Read the model definition and answer for the solid it produces. Units are mm, in the model's axes. A direction names the side the tool comes from. Give positions to 0.01 mm unless a question says otherwise; leave off trailing zeros. Loops run counter-clockwise (first coordinate to the right, second up) from the corner with the lowest first, then second, coordinate; pieces in that order, holes last.
(1) Find section A-A, the plane y = -16. Write down the section's boundary in (x, z), then the cut area to 3 significant figures.
(2) Find section B-B, the plane z = 2. Write down the section's boundary in (x, y).
(3) Determine the mould class of faces 1 (the face through (5, -5, 5)), 2 (the face through (-1, -10, 40)), 3 (the face through (-27, -20, 1)) for opening direction Z: pulls with the +Z half, pulls with the -Z half, needs draft (parallel to the pull), parting line crosses it, or undercut.
(4) Which of the six approach directions +Z, -Z, +X, -X, +Y, -Y give full straight-line access (tool end or side, diameter ignored) to faces 4 (the face through (-32, -5, -20)), 5 (the face through (-1, 0, 1))?
(5) Find section D-D, the plane y = -6.5. Write down the section's boundary in (x, z), then the cut area to 3 significant figures.
(6) Find section C-C, the plane x = -32. Write down the section's boundary in (y, z).
(7) This flat-tipped pin is pushed along its axis until it touches: P1, Ø2.5, axis at x = -33.5, z = -21.5, coming from the -Y side. Where does it stop, or does it pass through?
(8) Straight lines are drawn through the part: probe 1 along Z at (x, y) = (-32, -9); probe 2 along Z at (x, y) = (-4.5, -17.5); probe 3 along Z at (x, y) = (-0.5, -6.75). For each, find the intervals that lie inside material, in ascending order.
```python
from build123d import *

# Parameters (mm, degrees)
F0_W     = 80
F0_H     = 80
F1_DEPTH = 20
F2_R     = 4
F3_DEPTH = 15
F5_DEPTH = 10
F7_DEPTH = 5


with BuildPart() as f1:
    # F0 (on Front) → F1 (new body)
    with BuildSketch(Plane.XZ):
        Rectangle(F0_W, F0_H)
    extrude(amount=F1_DEPTH)

    # F2 (on face) → F3 (cut)
    with BuildSketch(Plane.XZ.offset(20)):
        with Locations((-32, 20)):
            Circle(F2_R)
        with Locations((-32, -20)):
            Circle(F2_R)
    extrude(amount=-F3_DEPTH, mode=Mode.SUBTRACT)

    # F4 (on face) → F5 (cut)
    with BuildSketch(Plane.XZ.offset(20)):
        with BuildLine():
            Line((-15, -25), (25, -25))
            ThreePointArc((25, -25), (32.071068, -22.071068), (35, -15))
            Line((35, -15), (35, 25))
            ThreePointArc((35, 25), (32.071068, 32.071068), (25, 35))
            Line((25, 35), (-15, 35))
            ThreePointArc((-15, 35), (-22.071068, 32.071068), (-25, 25))
            Line((-25, 25), (-25, -15))
            ThreePointArc((-25, -15), (-22.071068, -22.071068), (-15, -25))
        make_face()
    extrude(amount=-F5_DEPTH, mode=Mode.SUBTRACT)

    # F6 (on face) → F7 (cut)
    with BuildSketch(Plane.XZ.offset(10)):
        with BuildLine():
            Line((19, 25), (-9, 25))
            ThreePointArc((-9, 25), (-13.242641, 23.242641), (-15, 19))
            Line((-15, 19), (-15, -9))
            ThreePointArc((-15, -9), (-13.242641, -13.242641), (-9, -15))
            Line((-9, -15), (19, -15))
            ThreePointArc((19, -15), (23.242641, -13.242641), (25, -9))
            Line((25, -9), (25, 19))
            ThreePointArc((25, 19), (23.242641, 23.242641), (19, 25))
        make_face()
    extrude(amount=-F7_DEPTH, mode=Mode.SUBTRACT)


solid = f1.part
```
Entries:
1. outline: (-40, -40) - (40, -40) - (40, 40) - (-40, 40) - close; hole circle Ø8 at (-32, -20); hole circle Ø8 at (-32, 20); hole (-25, -15) arc R10 ccw to (-15, -25) - (25, -25) arc R10 ccw to (35, -15) - (35, 25) arc R10 ccw to (25, 35) - (-15, 35) arc R10 ccw to (-25, 25) - close
1. area: 2,790 mm2
2. outline: (-40, -20) - (-25, -20) - (-25, -10) - (-15, -10) - (-15, -5) - (25, -5) - (25, -10) - (35, -10) - (35, -20) - (40, -20) - (40, 0) - (-40, 0) - close
3. face 1: undercut
3. face 2: pulls with the +Z half
3. face 3: needs draft
4. face 4: -Y
4. face 5: +Z, -Z, +X, -X, +Y
5. outline: (-40, -40) - (40, -40) - (40, 40) - (-40, 40) - close; hole circle Ø8 at (-32, -20); hole circle Ø8 at (-32, 20); hole (-15, -9) arc R6 ccw to (-9, -15) - (19, -15) arc R6 ccw to (25, -9) - (25, 19) arc R6 ccw to (19, 25) - (-9, 25) arc R6 ccw to (-15, 19) - close
5. area: 4,730 mm2
6. outline: (-20, -40) - (0, -40) - (0, 40) - (-20, 40) - (-20, 24) - (-5, 24) - (-5, 16) - (-20, 16) - (-20, -16) - (-5, -16) - (-5, -24) - (-20, -24) - close
7. P1: stops at y = -5
8. probe 1: z = -40 to -24, -16 to 16, 24 to 40
8. probe 2: z = -40 to -25, 35 to 40
8. probe 3: z = -40 to -15, 25 to 40
